Autodesk Inventor part; units mm, degrees
ref_plane "YZ Plane" through (0, 0, 0) normal (1, 0, 0) x (0, 1, 0)
ref_plane "XZ Plane" through (0, 0, 0) normal (0, 1, 0) x (-1, 0, 0)
ref_plane "XY Plane" through (0, 0, 0) normal (0, 0, 1) x (1, 0, 0)
sketch "Sketch1" plane through (0, 0, 0) normal (0, 0, 1) x (1, 0, 0)
  circle A0 centre (0, 0) radius 194.5
  circle A1 centre (0, 0) radius 234.5
  dimension "d0" = 40
  dimension "d1" = 389
extrude "Extrusion1" add sketch "Sketch1" along normal blind 40
sketch "Sketch2" plane through (0, 0, 40) normal (0, 0, 1) x (1, 0, 0)
  circle A0 centre (0, 0) radius 234.5 construction
  circle A1 centre (0, 0) radius 194.5 construction
  line L0 (0, 234.5) -> (0, 194.5) construction
  circle A2 centre (0, 214.5) radius 6.25
  dimension "d4" = 12.5
extrude "Extrusion2" cut sketch "Sketch2" against normal through all
sketch "Sketch3" plane through (0, 0, 40) normal (0, 0, 1) x (1, 0, 0)
  circle A0 centre (0, 214.5) radius 6.25
  circle A1 centre (0, 214.5) radius 13.75
  point P0 (0, 0)
  dimension "d10" = 27.5
extrude "Extrusion3" cut sketch "Sketch3" against normal blind 11
pattern_circular "Circular Pattern1" count 8 over 360 about axis through (0, 0, 0) along (0, 0, 1) of "Extrusion2", "Extrusion3"
sketch "Sketch4" plane through (0, 0, 0) normal (0, 0, -1) x (-1, 0, 0)
  circle A0 centre (0, 0) radius 234.5
  circle A1 centre (0, 0) radius 239.5
  dimension "d13" = 5
extrude "Extrusion4" add sketch "Sketch4" against normal blind 10
equation "\"d1\" = Вал_ось_диаметр_КОРМА"
equation "\"d2\" = Барабан_толщина_посад_кольца"
properties part number "ДМФ 01 32 Барабан Опорное кольцо КОРМА"
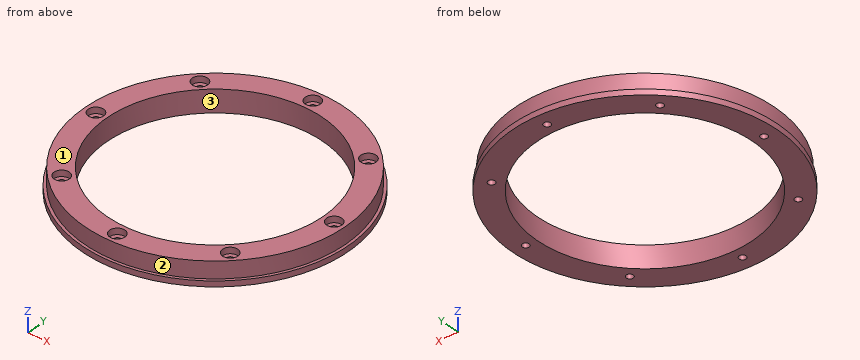
Can you work these out from the model? Positions are in its coordinate system, mm. Face numbers are marked on the shaded views. Give positions to 0.01 mm unless a question says otherwise; leave off trailing zeros. Loops run counter-clockwise (first coordinate to the right, second up) from the corner with the lowest first, then second, coordinate; pieces in that order, holes last. Notation, with made-up numbers: M -19.5,-37.75 L 8.5,-37.75 A17 cw 8.5,-31.75 Z; hole C 12,68 d7. An arc over 180 degrees is marked long. Answer in a Markdown table with one row per item.
1. Suppose I cut it at A-A on x = -214.5. Write out the boundary of the cut face in (y, z).
Taken from the geometry:
| item | result |
|---|---|
| outline | M -106.54,0 L -6.25,0 L -6.25,29 L -13.75,29 L -13.75,40 L -94.76,40 L -94.76,10 L -106.54,10 Z; M 6.25,0 L 106.54,0 L 106.54,10 L 94.76,10 L 94.76,40 L 13.75,40 L 13.75,29 L 6.25,29 Z |
2. If I drill on line 1 along Y through (x, z) = (0, 33); line 2 along Y through (x, z) = (152, 12); line 3 along X through (y, z) = (18, 24), over which ranges is the centre line in solid material (lowest first)?
Taken from the geometry:
| item | result |
|---|---|
| line 1 | y = -234.5 to -228.25, -200.75 to -194.5, 194.5 to 200.75, 228.25 to 234.5 |
| line 2 | y = -178.57 to -157.92, -145.43 to -121.35, 121.35 to 145.43, 157.92 to 178.57 |
| line 3 | x = -233.81 to -193.67, 193.67 to 233.81 |
3. Thinking about a two-plate mould opening in X: for the marked faces 1, 2 and 3, which applies, released by +X, released by -X, zero draft, split by the parting line, or undercut?
Taken from the geometry:
| item | result |
|---|---|
| face 1 | zero draft |
| face 2 | split by the parting line |
| face 3 | undercut |
4. Suppose I cut it at D-D on y = 38.5. Write out the boundary of the cut face in (x, z).
Taken from the geometry:
| item | result |
|---|---|
| outline | M -236.39,0 L -190.65,0 L -190.65,40 L -231.32,40 L -231.32,10 L -236.39,10 Z; M 190.65,0 L 236.39,0 L 236.39,10 L 231.32,10 L 231.32,40 L 190.65,40 Z |
5. For pin 1 Ø22 at (x, y) = (0, -214.5) entering from +Z; pin 2 Ø3 at (x, z) = (-112.5, 16.5) entering from +Y; pin 3 Ø3 at (y, z) = (191.5, 25.5) entering from -X, each with a flat end and sliding along its axis, tell me the tip position at first contact or that it passes through.
Taken from the geometry:
| item | result |
|---|---|
| pin 1 | stops at z = 29 |
| pin 2 | stops at y = 206.57 |
| pin 3 | stops at x = -137.44 |
6. Suppose I cut it at C-C on x = 101.5. Write out the boundary of the cut face in (y, z).
Taken from the geometry:
| item | result |
|---|---|
| outline | M -216.93,0 L -165.92,0 L -165.92,40 L -211.4,40 L -211.4,10 L -216.93,10 Z; M 165.92,0 L 216.93,0 L 216.93,10 L 211.4,10 L 211.4,40 L 165.92,40 Z |
